Geometry check sheet. Reference: drawing and pictorial views, mm from the part's lowest x, y, z. A direction names the side the tool comes from. Round coordinates to 2 decimals unless told otherwise and drop trailing zeros. Loops run counter-clockwise (first coordinate to the right, second up) from the corner with the lowest first, then second, coordinate; pieces in that order, holes last. Notation, with made-up numbers: M -35.5,22 L 17.5,22 A7 cw 17.5,29 Z; hole C 56.25,-7 d5. An arc over 180 degrees is marked long. One line per question, with ' | ' between items. Start each with the question number.
(1) Go/stop test with flat-tipped pins: P1, Ø12, axis at y = 26, z = 84, coming from the -X side; P2, Ø4, axis at x = 81.5, z = 28.5, coming from the +Y side; P3, Ø1.5, axis at x = 1.5, z = 94, coming from the +Y side. Record where each tip stops, or that it passes through.
(2) Section check A-A (x = 27.5). Record the boundary of the cut face in (y, z), and give its area (3 significant figures).
(3) Tool access check on the marked faces 1 and 2. Record the directions out of +Z, -Z, +X, -X, +Y, -Y that give a thin tool (end or side, any length) a straight path to the whole face; none if there is none.
(4) Thickness scan on probe 1 along Z at (x, y) = (27.5, 26); probe 2 along X at (y, z) = (39.5, 33); probe 3 along X at (y, z) = (36, 81). Record the ranges inside material, lowest first. Write a range as [from, to].
(5) Section check C-C (y = 41). Record the boundary of the cut face in (x, z), and give its area (3 significant figures).
(6) Section check B-B (z = 15.5). Record the boundary of the cut face in (x, y), and give its area (4 significant figures).
(7) Draft check along X on the marked faces 3, 4 and 5. Enter one of: +X half, -X half, draft (parallel to the pull), parting line (faces both ways), or undercut.
(8) Section check D-D (y = 9.5). Record the boundary of the cut face in (x, z), and give its area (3 significant figures).
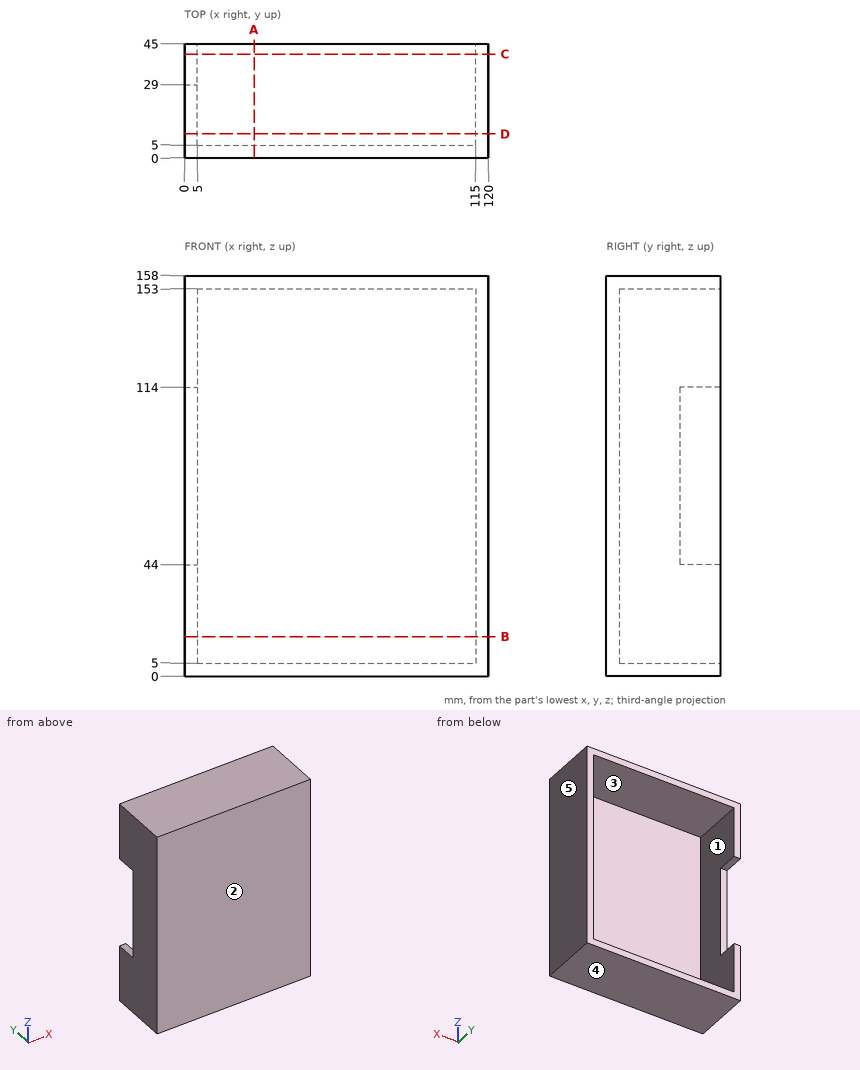
The answers:
1) P1: x = 0 | P2: y = 5 | P3: y = 29
2) outline: M 0,0 L 45,0 L 45,5 L 5,5 L 5,153 L 45,153 L 45,158 L 0,158 Z | area: 1,190 mm²
3) face 1: +Y | face 2: +Z, -Z, +X, -X, -Y
4) probe 1: [0, 5], [153, 158] | probe 2: [0, 5], [115, 120] | probe 3: [115, 120]
5) outline: M 0,0 L 120,0 L 120,158 L 0,158 L 0,114 L 5,114 L 5,153 L 115,153 L 115,5 L 5,5 L 5,44 L 0,44 Z | area: 2,330 mm²
6) outline: M 0,0 L 120,0 L 120,45 L 115,45 L 115,5 L 5,5 L 5,45 L 0,45 Z | area: 1,000 mm²
7) face 3: undercut | face 4: draft | face 5: +X half
8) outline: M 0,0 L 120,0 L 120,158 L 0,158 Z; hole M 5,5 L 115,5 L 115,153 L 5,153 Z | area: 2,680 mm²
